Read the model definition and answer for the solid it produces. Units are mm, in the model's axes. Round coordinates to 2 decimals unless told otherwise and drop trailing zeros. Write each loop counter-clockwise with the first axis right and the second up, starting at its lowest first coordinate (ties: lowest second). Pieces come first, ordered by that corner, then holes. Notation, with made-up numbers: (86.5, -33.75) - (108.5, -33.75) arc R21 ccw to (108.5, -9.75) - close; hole circle Ø1 at (32.5, 62.5). An arc over 180 degrees is marked (long way). One line per item, written item: value. Start each with the question number.
(1) Flat-ended cylindrical pins translate along their axes: pin 1 Ø5 at (x, y) = (129, -0.5) entering from -Z; pin 2 Ø4 at (y, z) = (-2.5, 5) entering from +X; pin 3 Ø5 at (x, y) = (143.5, -0.5) entering from +Z. Find the tip coordinate at first contact, or state that the pin passes through.
(2) A cutting plane is placed at B-B, the plane x = 247. Determine the outline of the cut face in (y, z), plus the area to 3 significant figures.
(3) Find the intervals of material crossed by L1, parallel to Z at x = 220, y = -5.5, in increasing order.
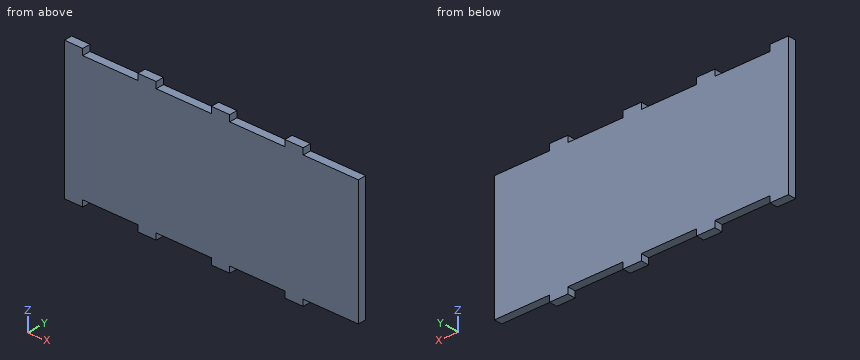
from build123d import *

# Parameters (mm, degrees)
SKETCH1_W                  = 359.0798
SKETCH1_H                  = 152.4
BOSS_EXTRUDE1_DEPTH        = 2.54
SKETCH2_W                  = 22.4424875
SKETCH2_H                  = 7.62
BOSS_EXTRUDE2_DEPTH        = 2.54
CONVERT_SOLID1_OUTLINE_W   = 7.46
CONVERT_SOLID1_OUTLINE_H   = 152.4
CONVERT_SOLID1_DEPTH       = 359.0798
CONVERT_SOLID1_2_OUTLINE_W = 7.46
CONVERT_SOLID1_2_OUTLINE_H = 7.62
CONVERT_SOLID1_2_DEPTH     = 22.4424875
CONVERT_SOLID1_START       = 89.76995
CONVERT_SOLID1_3_OUTLINE_W = 7.46
CONVERT_SOLID1_3_OUTLINE_H = 7.62
CONVERT_SOLID1_3_DEPTH     = 22.4424875
CONVERT_SOLID1_START_2     = 179.5399
CONVERT_SOLID1_4_OUTLINE_W = 7.46
CONVERT_SOLID1_4_OUTLINE_H = 7.62
CONVERT_SOLID1_4_DEPTH     = 22.4424875
CONVERT_SOLID1_START_3     = 269.30985
CONVERT_SOLID1_5_OUTLINE_W = 7.46
CONVERT_SOLID1_5_OUTLINE_H = 7.62
CONVERT_SOLID1_5_DEPTH     = 22.4424875


# Read off the part's stored shape, not the designer's step: Convert-Solid1
with BuildPart() as part:
    # Sketch1 → Boss-Extrude1 (new body)
    with BuildSketch(Plane(origin=(0, 0, 0), x_dir=(1, 0, 0), z_dir=(0, 1, 0))):
        with Locations((179.5399, 76.2)):
            Rectangle(SKETCH1_W, SKETCH1_H)
    extrude(amount=BOSS_EXTRUDE1_DEPTH)

    # Sketch2 → Boss-Extrude2 (add)
    with BuildSketch(Plane(origin=(0, 2.54, 0), x_dir=(1, 0, 0), z_dir=(0, 1, 0))):
        with Locations((11.22124375, 156.21)):
            Rectangle(SKETCH2_W, SKETCH2_H)
        with Locations((100.99119375, 156.21)):
            Rectangle(SKETCH2_W, SKETCH2_H)
        with Locations((190.76114375, 156.21)):
            Rectangle(SKETCH2_W, SKETCH2_H)
        with Locations((280.53109375, 156.21)):
            Rectangle(SKETCH2_W, SKETCH2_H)
        with Locations((11.22124375, -3.81)):
            Rectangle(SKETCH2_W, SKETCH2_H)
        with Locations((100.99119375, -3.81)):
            Rectangle(SKETCH2_W, SKETCH2_H)
        with Locations((190.76114375, -3.81)):
            Rectangle(SKETCH2_W, SKETCH2_H)
        with Locations((280.53109375, -3.81)):
            Rectangle(SKETCH2_W, SKETCH2_H)
    extrude(amount=-BOSS_EXTRUDE2_DEPTH)

    # Convert-Solid1 outline → Convert-Solid1 (add)
    with BuildSketch(Plane.YZ):
        with Locations((-3.73, -76.2)):
            Rectangle(CONVERT_SOLID1_OUTLINE_W, CONVERT_SOLID1_OUTLINE_H)
    extrude(amount=CONVERT_SOLID1_DEPTH)

    # Convert-Solid1 2 outline → Convert-Solid1 2 (add)
    with BuildSketch(Plane.YZ):
        with Locations((-3.73, 3.81)):
            Rectangle(CONVERT_SOLID1_2_OUTLINE_W, CONVERT_SOLID1_2_OUTLINE_H)
        with Locations((-3.73, -156.21)):
            Rectangle(CONVERT_SOLID1_2_OUTLINE_W, CONVERT_SOLID1_2_OUTLINE_H)
    extrude(amount=CONVERT_SOLID1_2_DEPTH)

    # Convert-Solid1 3 outline → Convert-Solid1 3 (add)
    with BuildSketch(Plane.YZ.offset(CONVERT_SOLID1_START)):
        with Locations((-3.73, 3.81)):
            Rectangle(CONVERT_SOLID1_3_OUTLINE_W, CONVERT_SOLID1_3_OUTLINE_H)
        with Locations((-3.73, -156.21)):
            Rectangle(CONVERT_SOLID1_3_OUTLINE_W, CONVERT_SOLID1_3_OUTLINE_H)
    extrude(amount=CONVERT_SOLID1_3_DEPTH)

    # Convert-Solid1 4 outline → Convert-Solid1 4 (add)
    with BuildSketch(Plane.YZ.offset(CONVERT_SOLID1_START_2)):
        with Locations((-3.73, 3.81)):
            Rectangle(CONVERT_SOLID1_4_OUTLINE_W, CONVERT_SOLID1_4_OUTLINE_H)
        with Locations((-3.73, -156.21)):
            Rectangle(CONVERT_SOLID1_4_OUTLINE_W, CONVERT_SOLID1_4_OUTLINE_H)
    extrude(amount=CONVERT_SOLID1_4_DEPTH)

    # Convert-Solid1 5 outline → Convert-Solid1 5 (add)
    with BuildSketch(Plane.YZ.offset(CONVERT_SOLID1_START_3)):
        with Locations((-3.73, 3.81)):
            Rectangle(CONVERT_SOLID1_5_OUTLINE_W, CONVERT_SOLID1_5_OUTLINE_H)
        with Locations((-3.73, -156.21)):
            Rectangle(CONVERT_SOLID1_5_OUTLINE_W, CONVERT_SOLID1_5_OUTLINE_H)
    extrude(amount=CONVERT_SOLID1_5_DEPTH)


solid = part.part
Here are the results:
1. pin 1: z = -152.4
1. pin 2: x = 291.75
1. pin 3: z = 0
2. outline: (-7.46, -152.4) - (2.54, -152.4) - (2.54, 0) - (-7.46, 0) - close
2. area: 1,520 mm²
3. L1: -152.4 to 0
